The listing builds one solid part. Answer for the finished solid, in the listing's coordinates (mm). A direction names the side the tool comes from. Round coordinates to 2 decimals unless told otherwise and drop trailing zeros. Order: outer loops, then holes, each group sorted by start corner. A loop starts at its lowest first (then second) coordinate and runs counter-clockwise, first axis right, second up. Notation, with made-up numbers: (53, -29.75) - (65, -29.75) arc R23 ccw to (65, -12.75) - close; hole circle Ø3 at (15, 50). An arc over 180 degrees is marked (long way). Write item = value, one per line.
from build123d import *

# Parameters (mm, degrees)
CUT_EXTRUDE1_DEPTH      = 76.475058221
CUT_EXTRUDE1_DEPTH_BACK = 76.475058221
SKETCH2_R               = 1.653940434


with BuildPart() as part:
    # Sketch1 → Revolve1 (revolve)
    with BuildSketch(Plane.XY, mode=Mode.PRIVATE) as revolve1_sk:
        Polygon((0, 0), (4.953, 0), (4.953, -14.6812), (6.6929, -14.6812), (6.6929, -34.671), (5.5753, -34.671), (5.5753, -51.5112), (2.3114, -74.8792), (0, -74.8792), align=None)
    revolve(revolve1_sk.sketch.rotate(Axis((0, -74.8792, 0), (0, 1, 0)), 90), axis=Axis((0, -74.8792, 0), (0, 1, 0)))

    # Sketch2 → Cut-Extrude1 (cut, two sides: drawn at the far end of the back side and taken through both)
    with BuildSketch(Plane.XY.offset(-CUT_EXTRUDE1_DEPTH_BACK)):
        with Locations((0, -39.751)):
            Circle(SKETCH2_R)
    extrude(amount=CUT_EXTRUDE1_DEPTH + CUT_EXTRUDE1_DEPTH_BACK, mode=Mode.SUBTRACT)


solid = part.part
Q1. Determine the mould class of faces 1 (the face through (-0.22, -38.11, -0.08)), 2 (the face through (0, 0, 0)), 3 (the face through (-1.488, -7.443, -4.724)) for opening direction Y: released by +Y, released by -Y, zero draft, split by the parting line, or undercut.
Model answer:
face_1 = undercut
face_2 = released by +Y
face_3 = zero draft
Q2. Section C-C on y = -37 is taken. Determine the outline of the cut face in (x, z), then the cut area to 3 significant figures.
Model answer:
outline = circle Ø11.15 at (0, 0)
area = 97.7 mm^2
Q3. Section A-A on x = 0 is taken. Determine the outline of the cut face in (y, z), then the cut area to 3 significant figures.
Model answer:
outline = (-74.88, -2.31) - (-51.51, -5.58) - (-41.4, -5.58) - (-41.4, 5.58) - (-51.51, 5.58) - (-74.88, 2.31) - close; (-38.1, -5.58) - (-34.67, -5.58) - (-34.67, -6.69) - (-14.68, -6.69) - (-14.68, -4.95) - (0, -4.95) - (0, 4.95) - (-14.68, 4.95) - (-14.68, 6.69) - (-34.67, 6.69) - (-34.67, 5.58) - (-38.1, 5.58) - close
area = 748 mm^2
Q4. For faces 4 (the face through (0, -74.879, 0)), 5 (the face through (-2.5, -14.681, -4.5)), 6 (the face through (-1.67, -43.21, -5.32)), determine the directions among +Z, -Z, +X, -X, +Y, -Y from which every point of the face is accessible in a straight line to the end or side of a thin tool.
Model answer:
face_4 = +Z, -Z, +X, -X, -Y
face_5 = +Y
face_6 = -Y
Q5. Section B-B on z = 0 is taken. Determine the outline of the cut face in (x, y), then the cut area to 3 significant figures.
Model answer:
outline = (-6.69, -34.67) - (-5.58, -34.67) - (-5.58, -51.51) - (-2.31, -74.88) - (2.31, -74.88) - (5.58, -51.51) - (5.58, -34.67) - (6.69, -34.67) - (6.69, -14.68) - (4.95, -14.68) - (4.95, 0) - (-4.95, 0) - (-4.95, -14.68) - (-6.69, -14.68) - close; hole circle Ø3.31 at (0, -39.75)
area = 776 mm^2
Q6. Find the intervals of material crossed by line 1 (Y direction, x = 0, z = -1.25); line 2 (Y direction, x = 6, z = -1); line 3 (X direction, y = -43.5, z = 1), in increasing order. Write a range as from..to.
Model answer:
line_1 = -74.88..-41.4, -38.1..0
line_2 = -34.67..-14.68
line_3 = -5.48..5.48
Q7. Flat-ended cylindrical pins translate along their axes: P1, Ø1, axis at x = 3, y = -34.5, coming from the -Z side; P2, Ø3, axis at x = 1, y = -50, coming from the -Z side; P3, Ø5, axis at x = 1.5, z = -4.5, coming from the -Y side; P4, Ø3, axis at x = -5, y = -42.5, coming from the -Z side. Find the tip coordinate at first contact, or state that the pin passes through.
Model answer:
P1 = -6.21
P2 = -5.58
P3 = -74.88
P4 = -4.34
Q8. Section D-D on y = -5.5 is taken. Determine the outline of the cut face in (x, z).
Model answer:
outline = circle Ø9.91 at (0, 0)
